```python
from build123d import *

# Parameters (mm, degrees)
F0_R      = 20
F1_DEPTH  = 17
F2_R      = 9.5
F3_DEPTH  = 13
F2_R_2    = 10.5
F4_DEPTH  = 0.25
F5_R      = 2
F6_DEPTH  = 25
F7_R      = 4.25
F8_DEPTH  = 2
F9_R      = 2.5
F10_DEPTH = 2
F11_R     = 0.5
F12_DEPTH = 1


# Not quite as in the source:
# - a feature names something its author has since deleted; it is built from what else it names


with BuildPart() as f1:
    # F0 (on Front) → F1 (new body)
    with BuildSketch(Plane.XZ):
        Circle(F0_R)
    extrude(amount=F1_DEPTH)

    # F2 (on face) → F3 (cut)
    with BuildSketch(Plane.XZ.offset(17)):
        Circle(F2_R)
    extrude(amount=-F3_DEPTH, mode=Mode.SUBTRACT)

    # F2 (on face) → F4 (join)
    with BuildSketch(Plane.XZ.offset(17)):
        Circle(F2_R_2)
        Circle(F2_R, mode=Mode.SUBTRACT)
    extrude(amount=F4_DEPTH)

    # F5 (on face) → F6 (cut)
    with BuildSketch(Plane.XZ.offset(4)):
        with Locations((0, 6.7485035397)):
            Circle(F5_R)
        with Locations((4.7719126158, 4.7719126158)):
            Circle(F5_R)
        with Locations((6.7485035397, 0)):
            Circle(F5_R)
        with Locations((4.7719126158, -4.7719126158)):
            Circle(F5_R)
        with Locations((0, -6.7485035397)):
            Circle(F5_R)
        with Locations((-4.7719126158, -4.7719126158)):
            Circle(F5_R)
        with Locations((-6.7485035397, 0)):
            Circle(F5_R)
        with Locations((-4.7719126158, 4.7719126158)):
            Circle(F5_R)
    extrude(amount=-F6_DEPTH, mode=Mode.SUBTRACT)

    # F7 (on face) → F8 (join)
    with BuildSketch(Plane.XZ.offset(4)):
        Circle(F7_R)
    extrude(amount=F8_DEPTH)

    # F9 (on face) → F10 (join)
    with BuildSketch(Plane.XZ.offset(6)):
        Circle(F9_R)
    extrude(amount=F10_DEPTH)

    # F11 (on face) → F12 (join)
    with BuildSketch(Plane.XZ.offset(6)):
        with Locations((0, 3.2268003561)):
            Circle(F11_R)
        with Locations((1.8966656614, 2.6105363255)):
            Circle(F11_R)
        with Locations((3.0688695054, -0.9971361475)):
            Circle(F11_R)
        with Locations((3.0688695054, 0.9971361475)):
            Circle(F11_R)
        with Locations((1.8966656614, -2.6105363255)):
            Circle(F11_R)
        with Locations((0, -3.2268003561)):
            Circle(F11_R)
        with Locations((-1.8966656614, -2.6105363255)):
            Circle(F11_R)
        with Locations((-3.0688695054, -0.9971361475)):
            Circle(F11_R)
        with Locations((-3.0688695054, 0.9971361475)):
            Circle(F11_R)
        with Locations((-1.8966656614, 2.6105363255)):
            Circle(F11_R)
    extrude(amount=F12_DEPTH)


solid = f1.part
```
Input: part model. Units: mm. Frame: model coordinates. A direction names the side the tool comes from. Coordinates: 2 decimals unless noted, no trailing zeros. Write each loop counter-clockwise with the first axis right and the second up, starting at its lowest first coordinate (ties: lowest second). Pieces come first, ordered by that corner, then holes. Notation, with made-up numbers: (19.25, 36) - (64.25, 36) arc R13 ccw to (64.25, 42) - close; hole circle Ø9 at (43, 25). An arc over 180 degrees is marked (long way). Put each result on its own line as item: value. Start each with the question number.
1) Cut plane A-A (x = -7.5). Return the cut outline in (y, z), plus the area to 3 significant figures.
2) Ray query, L1, parallel to Z at x = 0, y = -12.5; L2, parallel to Z at x = 5.5, y = -3.25; L3, parallel to X at y = -1, z = -6.5. Return the intervals inside material, ascending.
3) Contact query for flat-ended pins moving along their axis: pin 1 (10 mm diameter, centred on x = -15.5, y = -7, fed in from +Z); pin 2 (2 mm diameter, centred on x = -9.5, y = -12, fed in from -Z); pin 3 (1.1 mm diameter, centred on x = 3, z = 1, fed in from -Y); pin 4 (2.5 mm diameter, centred on x = 4.77, z = -4.77, fed in from -Y). Output: stop coordinate, or through.
4) Cut plane C-C (z = 0). Return the cut outline in (x, y).
5) Cut plane B-B (y = -6.5). State how many separate pieces and enclosed holes the cut face has, plus the area to 3 significant figures.
6) Mould query, pull axis Z, two halves, no side actions, for faces 3 (the face through (-5, -17.25, -9)), 4 (the face through (3, -7, 1)). Classes: pulls with the +Z half, pulls with the -Z half, needs draft (parallel to the pull), parting line crosses it, or undercut.
7) Cut plane D-D (y = -13.25). Return the cut outline in (x, z).
8) Reachability of faces 1 (the face through (4.512, -2.028, 6.755)), 2 (the face through (-1.962, -6.493, -2.115)) from +Z, -Z, +X, -X, +Y, -Y: full face, straight path, thin tool, end or side. Return the list, or none.
Resolved:
1. outline: (-17.25, -7.35) - (-17, -7.35) - (-17, -18.54) - (0, -18.54) - (0, -1.85) - (-4, -1.85) - (-4, -5.83) - (-17.25, -5.83) - close; (-17.25, 5.83) - (-4, 5.83) - (-4, 1.85) - (0, 1.85) - (0, 18.54) - (-17, 18.54) - (-17, 7.35) - (-17.25, 7.35) - close
1. area: 465 mm2
2. L1: z = -20 to -9.5, 9.5 to 20
2. L2: z = -19.23 to -6.63, -2.91 to -1.56, 1.56 to 2.91, 6.63 to 19.23
2. L3: x = -18.91 to -5.78, -3.77 to -1.98, 1.98 to 3.77, 5.78 to 18.91
3. pin 1: stops at z = 17.02
3. pin 2: stops at z = -18.1
3. pin 3: stops at y = -7
3. pin 4: passes through
4. outline: (-20, -17) - (-10.5, -17) - (-10.5, -17.25) - (-9.5, -17.25) - (-9.5, -4) - (-8.75, -4) - (-8.75, 0) - (-20, 0) - close; (-4.75, -4) - (-4.25, -4) - (-4.25, -6) - (-2.5, -6) - (-2.5, -8) - (2.5, -8) - (2.5, -6) - (4.25, -6) - (4.25, -4) - (4.75, -4) - (4.75, 0) - (-4.75, 0) - close; (8.75, -4) - (9.5, -4) - (9.5, -17.25) - (10.5, -17.25) - (10.5, -17) - (20, -17) - (20, 0) - (8.75, 0) - close
5. separate pieces: 12
5. enclosed holes: 1
5. area: 1,000 mm2
6. face 3: needs draft
6. face 4: undercut
7. outline: circle Ø40 at (0, 0); hole circle Ø19 at (0, 0)
8. face 1: +Y, -Y
8. face 2: -Y
